Autodesk Inventor part; units mm, degrees
ref_plane "YZ Plane" through (0, 0, 0) normal (1, 0, 0) x (0, 1, 0)
ref_plane "XZ Plane" through (0, 0, 0) normal (0, 1, 0) x (-1, 0, 0)
ref_plane "XY Plane" through (0, 0, 0) normal (0, 0, 1) x (1, 0, 0)
sketch "Sketch1" plane through (0, 0, 0) normal (0, 0, 1) x (1, 0, 0)
  line L0 (0, 0) -> (25.4, 0)
  line L1 (25.4, 0) -> (25.4, 25.4)
  line L2 (25.4, 25.4) -> (0, 25.4)
  line L3 (0, 25.4) -> (0, 0)
  circle A0 centre (12.7, 12.7) radius 3.175
  dimension "d0" = 25.4
  dimension "d1" = 25.4
  dimension "d2" = 6.35
  dimension "d7" = 12.7
  dimension "d8" = 12.7
extrude "Extrusion1" add sketch "Sketch1" along normal blind 609.6
sketch "Sketch2" plane through (0, 0, 609.6) normal (0, 0, 1) x (1, 0, 0)
  line L0 (25.4, 25.4) -> (0, 25.4)
  line L1 (0, 25.4) -> (0, 0)
  circle A0 centre (12.7, 12.7) radius 3.175
  line L2 (0, 0) -> (25.4, 0)
  line L3 (25.4, 0) -> (25.4, 25.4)
  line L4 (25.4, 25.4) -> (0, 25.4)
  line L5 (0, 25.4) -> (0, 0)
  line L6 (12.7, 19.05) -> (9.525, 19.05)
  line L7 (9.525, 19.05) -> (15.875, 19.05)
  line L8 (15.875, 19.05) -> (19.05, 25.4)
  line L9 (9.525, 19.05) -> (6.35, 25.4)
  dimension "d13" = 6.35
  dimension "d14" = 6.35
  dimension "d15" = 3.175
  dimension "d16" = 6.35
fillet "Fillet1" radius 1.5875 4 edges at (25.4, 25.4, 304.8) (0, 25.4, 304.8) (25.4, 0, 304.8) (0, 0, 304.8)
extrude "Extrusion2" cut sketch "Sketch2" against normal blind 609.6 contours L8 L7 L6 L9 L0
pattern_circular "Circular Pattern1" count 4 over 360 about axis through (12.7, 12.7, 0) along (0, 0, 1) of "Extrusion2"
sketch "Sketch3" plane through (0, 0, 609.6) normal (0, 0, 1) x (1, 0, 0)
  line L0 (19.05, 15.875) -> (25.4, 19.05)
  line L1 (25.4, 19.05) -> (25.4, 23.8125)
  arc A0 (25.4, 23.8125) -> (23.8125, 25.4) centre (23.8125, 23.8125) ccw
  line L2 (23.8125, 25.4) -> (19.05, 25.4)
  line L3 (19.05, 25.4) -> (15.875, 19.05)
  line L4 (15.875, 19.05) -> (9.525, 19.05)
  line L5 (9.525, 19.05) -> (6.35, 25.4)
  line L6 (6.35, 25.4) -> (1.5875, 25.4)
  arc A1 (1.5875, 25.4) -> (0, 23.8125) centre (1.5875, 23.8125) ccw
  line L7 (0, 23.8125) -> (0, 19.05)
  line L8 (0, 19.05) -> (6.35, 15.875)
  line L9 (6.35, 15.875) -> (6.35, 9.525)
  line L10 (6.35, 9.525) -> (0, 6.35)
  line L11 (0, 6.35) -> (0, 1.5875)
  arc A2 (0, 1.5875) -> (1.5875, 0) centre (1.5875, 1.5875) ccw
  line L12 (1.5875, 0) -> (6.35, 0)
  line L13 (6.35, 0) -> (9.525, 6.35)
  line L14 (9.525, 6.35) -> (15.875, 6.35)
  line L15 (15.875, 6.35) -> (19.05, 0)
  line L16 (19.05, 0) -> (23.8125, 0)
  arc A3 (23.8125, 0) -> (25.4, 1.5875) centre (23.8125, 1.5875) ccw
  line L17 (25.4, 1.5875) -> (25.4, 6.35)
  line L18 (25.4, 6.35) -> (19.05, 9.525)
  line L19 (19.05, 9.525) -> (19.05, 15.875)
  circle A4 centre (12.7, 12.7) radius 3.175
  point P0 (0, 0)
extrude "Extrusion3" cut sketch "Sketch3" against normal blind 517.525
sketch "Sketch4" plane through (0, 0, 92.075) normal (0, 0, 1) x (1, 0, 0)
  circle A0 centre (12.7, 12.7) radius 3.175
  line L0 (25.4, 19.05) -> (19.05, 15.875)
  line L1 (25.4, 23.8125) -> (25.4, 19.05)
  arc A1 (25.4, 23.8125) -> (23.8125, 25.4) centre (23.8125, 23.8125) ccw
  line L2 (19.05, 25.4) -> (23.8125, 25.4)
  line L3 (15.875, 19.05) -> (19.05, 25.4)
  line L4 (9.525, 19.05) -> (15.875, 19.05)
  line L5 (6.35, 25.4) -> (9.525, 19.05)
  line L6 (1.5875, 25.4) -> (6.35, 25.4)
  arc A2 (1.5875, 25.4) -> (0, 23.8125) centre (1.5875, 23.8125) ccw
  line L7 (0, 19.05) -> (0, 23.8125)
  line L8 (6.35, 15.875) -> (0, 19.05)
  line L9 (6.35, 9.525) -> (6.35, 15.875)
  line L10 (0, 6.35) -> (6.35, 9.525)
  line L11 (0, 1.5875) -> (0, 6.35)
  arc A3 (0, 1.5875) -> (1.5875, 0) centre (1.5875, 1.5875) ccw
  line L12 (6.35, 0) -> (1.5875, 0)
  line L13 (9.525, 6.35) -> (6.35, 0)
  line L14 (15.875, 6.35) -> (9.525, 6.35)
  line L15 (19.05, 0) -> (15.875, 6.35)
  line L16 (23.8125, 0) -> (19.05, 0)
  arc A4 (23.8125, 0) -> (25.4, 1.5875) centre (23.8125, 1.5875) ccw
  line L17 (25.4, 6.35) -> (25.4, 1.5875)
  line L18 (19.05, 9.525) -> (25.4, 6.35)
  line L19 (19.05, 15.875) -> (19.05, 9.525)
  point P0 (0, 0)
extrude "Extrusion4" cut sketch "Sketch4" against normal blind 6.35
properties part number "Mock 8020 3.375in" material "Aluminum 6061"
Check sheet for the modelled part. Datum: model origin and axes. Units: mm. A direction names the side the tool comes from. Give positions to 0.01 mm unless a question says otherwise; leave off trailing zeros. Loops run counter-clockwise (first coordinate to the right, second up) from the corner with the lowest first, then second, coordinate; pieces in that order, holes last. Notation, with made-up numbers: M 12,74.5 L 17,74.5 A28 cw 17,94.5 Z; hole C -4,-4.75 d5. An arc over 180 degrees is marked long. Answer as a JSON object with one key per item and string values. Group by question number.
Q1. Material ranges on line 1 along Y through (x, z) = (12.7, 21) (3 decimals); line 2 along X through (y, z) = (12.5, 18.5); line 3 along Y through (x, z) = (24.5, 21.5), recorded low to high. Write a range as [from, to].
Q2. Cross-section at D-D on y = 8.5. Record the cut outline in (x, z) (3 decimals), then the cut area to 3 significant figures.
Q3. Access from +Z, -Z, +X, -X, +Y, -Y to the whole of each face (thin tool, end or side, straight path). Record for faces 4 (the flat face through (7.96, 22.18, 43.46)), 5 (the flat face through (7.96, 3.22, 43.46)), 6 (the flat face through (6.35, 13, 43)).
Q4. Go/stop test with flat-tipped pins: P1, Ø7, axis at y = 12, z = 26.5, coming from the -X side; P2, Ø7, axis at x = 13.5, z = 42, coming from the +Y side; P3, Ø5, axis at y = 11.5, z = 39.5, coming from the +X side; P4, Ø2, axis at x = 14, y = 4, coming from the +Z side. Record where each tip stops, or that it passes through.
Q5. Release check for a two-part mould opening along X. For faces 1 (the cylindrical face through (24.92, 0.45, 43.46)), 2 (the flat face through (17.44, 22.18, 43.46)), 3 (the flat face through (10, 16, 0)) record: released by +X, released by -X, zero draft, split by the parting line, or undercut.
Q6. Cross-section at A-A on x = 12.7. Record the cut outline in (y, z) (3 decimals), then the cut area to 3 significant figures.
Evaluation:
{
 "1": {"line 1": "y = [6.35, 9.525], [15.875, 19.05]", "line 2": "x = [6.35, 9.53], [15.87, 19.05]", "line 3": "y = [0.16, 6.8], [18.6, 25.24]"},
 "2": {"outline": "M 4.3,0 L 21.1,0 L 21.1,85.725 L 4.3,85.725 Z", "area": "1,440 mm2"},
 "3": {"face 4": "+Z, -Z, +Y", "face 5": "+Z, -Z, -Y", "face 6": "+Z, -Z, -X"},
 "4": {"P1": "stops at x = 4.3", "P2": "stops at y = 21.3", "P3": "stops at x = 20.1", "P4": "passes through"},
 "5": {"face 1": "released by +X", "face 2": "undercut", "face 3": "zero draft"},
 "6": {"outline": "M 6.35,0 L 9.525,0 L 9.525,85.725 L 6.35,85.725 Z; M 15.875,0 L 19.05,0 L 19.05,85.725 L 15.875,85.725 Z", "area": "544 mm2"}
}
